CAD build for the part. Positions are in the model's coordinates, mm. A direction names the side the tool comes from. Round coordinates to 2 decimals unless told otherwise and drop trailing zeros. Write each loop counter-clockwise with the first axis right and the second up, starting at its lowest first coordinate (ties: lowest second). Pieces come first, ordered by that corner, then holes. Notation, with made-up numbers: (75, 14.5) - (87, 14.5) arc R21 ccw to (87, 22.5) - close; hole circle Ø5 at (41.25, 38.5). An arc over 180 degrees is marked (long way). Answer in a Markdown table with one row per item.
```python
from build123d import *

# Parameters (mm, degrees)
SCALE1_SCALE = 1.142857143
SCALE2_SCALE = 0.997091816


with BuildPart() as part:
    # Sketch1 → Revolve1 (revolve)
    with BuildSketch(Plane.XY, mode=Mode.PRIVATE) as revolve1_sk:
        Polygon((0, 7), (-0.5, 7), (-0.5, 8), (-5.1, 8), (-5.1, 9.5), (-4.068629558, 10.531370442), (0, 10.531370442), align=None)
    revolve1 = revolve(revolve1_sk.sketch.rotate(Axis((0, 0, 0), (-1, 0, 0)), 90), axis=Axis((0, 0, 0), (-1, 0, 0)))

    # Mirror1: Revolve1 across plane
    add(revolve1.mirror(Plane(origin=(0, 10.531370442, 0), x_dir=(0, 0, 1), z_dir=(1, 0, 0))))


with BuildPart() as part_1:
    # Scale1: scaled about (0, 0, 0)
    add(part.part.scale(SCALE1_SCALE))


with BuildPart() as part_2:
    # Scale2: scaled about (0, 0, 0)
    add(part_1.part.scale(SCALE2_SCALE))


solid = part_2.part
```
Q1. Saw through at C-C on x = 1.5. List the corners of the cut face in (y, z).
Computed:
| item | result |
|---|---|
| outline | circle Ø24 at (0, 0); hole circle Ø18.23 at (0, 0) |
Q2. 3-axis set-ups, long thin cutter, end or side, ignore diameter. For faces 1 (the flat face through (-5.812, 8, -5)), 2 (the flat face through (-0.57, 7, 5)), 3 (the flat face through (0.57, 7, 5)): which of +Z, -Z, +X, -X, +Y, -Y reach the whole face in a straight line?
Computed:
| item | result |
|---|---|
| face 1 | +Z, -Z, -X, +Y, -Y |
| face 2 | -X |
| face 3 | +X |
Q3. Pull direction Y, two halves, no side cores. Call faces 4 (the flat face through (5.812, 8, -5)), 5 (the cylindrical face through (-3.227, -2.738, -8.695)), 6 (the conical face through (-5.7, 4.2, -10.1)): released by +Y, released by -Y, zero draft, split by the parting line, or undercut.
Computed:
| item | result |
|---|---|
| face 4 | zero draft |
| face 5 | undercut |
| face 6 | split by the parting line |
Q4. Drill centre lines: line 1 (Y direction, x = -0.2, z = 0); line 2 (Y direction, x = -2.25, z = 0); line 3 (X direction, y = 8, z = 2.25). Where is each one in solid material? Low to high.
Computed:
| item | result |
|---|---|
| line 1 | y = -12 to -7.98, 7.98 to 12 |
| line 2 | y = -12 to -9.12, 9.12 to 12 |
| line 3 | x = -0.57 to 0.57 |
Q5. Saw through at A-A on z = 0. List the corners of the cut face in (x, y), then the cut area to 3 significant figures.
Computed:
| item | result |
|---|---|
| outline | (-5.81, -10.83) - (-4.64, -12) - (4.64, -12) - (5.81, -10.83) - (5.81, -9.12) - (0.57, -9.12) - (0.57, -7.98) - (-0.57, -7.98) - (-0.57, -9.12) - (-5.81, -9.12) - close; (-5.81, 9.12) - (-0.57, 9.12) - (-0.57, 7.98) - (0.57, 7.98) - (0.57, 9.12) - (5.81, 9.12) - (5.81, 10.83) - (4.64, 12) - (-4.64, 12) - (-5.81, 10.83) - close |
| area | 66.9 mm2 |
Q6. Flat gauge pins, fed straight in: pin 1 (4 mm diameter, centred on x = 3.5, z = 6.5, fed in from -Y); pin 2 (8 mm diameter, centred on y = 6, z = -2, fed in from +X); pin 3 (1.5 mm diameter, centred on x = -4.5, z = 8.5, fed in from -Y); pin 4 (9.5 mm diameter, centred on y = 0, z = 0, fed in from -X). Where does each tip first touch, or does it go through?
Computed:
| item | result |
|---|---|
| pin 1 | stops at y = -11.13 |
| pin 2 | stops at x = 5.81 |
| pin 3 | stops at y = -9.16 |
| pin 4 | passes through |
